```python
from build123d import *


with BuildPart() as f1:
    # F0 (on Front) → F1 (revolve)
    with BuildSketch(Plane.XZ):
        with BuildLine():
            Line((0, 25), (0, 0))
            Line((0, 0), (6.25, 0))
            Line((6.25, 0), (6.25, 0.891346))
            ThreePointArc((6.25, 0.891346), (6.227951, 0.982633), (6.166667, 1.053793))
            ThreePointArc((6.166667, 1.053793), (5.75, 1.866025), (6.166667, 2.678258))
            ThreePointArc((6.166667, 2.678258), (6.227951, 2.749418), (6.25, 2.840705))
            Line((6.25, 2.840705), (6.25, 24))
            ThreePointArc((6.25, 24), (5.957107, 24.707107), (5.25, 25))
            Line((5.25, 25), (0, 25))
        make_face()
    revolve(axis=Axis((0, 0, 12.5), (0, 0, -1)))


solid = f1.part
```
For this review, take the finished solid that the model builds, in its own axes (mm). Round coordinates to 2 decimals unless told otherwise and drop trailing zeros. Order: outer loops, then holes, each group sorted by start corner. A loop starts at its lowest first (then second) coordinate and runs counter-clockwise, first axis right, second up.
Q1. Wall thickness on line 1 (X direction, y = -0.25, z = 20.25) (3 decimals); line 2 (Y direction, x = -2.5, z = 1.5); line 3 (Y direction, x = 1, z = 8): over which ranges is each line inside the solid? List them lowest first.
Findings below:
line 1: x = -6.245 to 6.245
line 2: y = -5.26 to 5.26
line 3: y = -6.17 to 6.17
Q2. We need section A-A, the plane z = 20.75. Give the boundary of the cut face in (x, y), plus the area to 3 significant figures.
Findings below:
outline: circle Ø12.5 at (0, 0)
area: 123 mm2
Q3. Insertion check: P1, Ø3, axis at y = -3, z = 18, coming from the -X side; P2, Ø1.5, axis at x = -2.5, z = 15.5, coming from the -Y side; P3, Ø1.5, axis at y = -4, z = 14, coming from the -X side. Each pin has a flat end and moves straight along its axis. Give the tip position at first contact, or say it passes through.
Findings below:
P1: stops at x = -6.07
P2: stops at y = -6
P3: stops at x = -5.34
